from build123d import *

# Parameters (mm, degrees)
SZKIC1_W                     = 53
SZKIC1_H                     = 374
SZKIC1_W_2                   = 24
SZKIC1_H_2                   = 365
DODANIE_WYCI_GNI_CIE2_DEPTH  = 12
SZKIC2_W                     = 12
SZKIC2_H                     = 3.5
WYTNIJ_WYCI_GNI_CIE1_DEPTH   = 2
SZKIC3_W                     = 53
SZKIC3_H                     = 374
DODANIE_WYCI_GNI_CIE3_DEPTH  = 2
SZKIC4_W                     = 13.3
SZKIC4_H                     = 30.500081729
SZKIC4_W_2                   = 9.4
SZKIC4_H_2                   = 64.96
WYTNIJ_WYCI_GNI_CIE2_DEPTH   = 2
SZKIC5_W                     = 2
SZKIC5_H                     = 374
DODANIE_WYCI_GNI_CIE4_DEPTH  = 43
DODANIE_WYCI_GNI_CIE5_DEPTH  = 41.5
SZKIC7_W                     = 25.5
SZKIC7_H                     = 38.500081729
DODANIE_WYCI_GNI_CIE6_DEPTH  = 1.5
DODANIE_WYCI_GNI_CIE7_DEPTH  = 43
DODANIE_WYCI_GNI_CIE8_DEPTH  = 43
SZKIC15_W                    = 57
SZKIC15_H                    = 374
DODANIE_WYCI_GNI_CIE10_DEPTH = 1
SZKIC16_W                    = 57
SZKIC16_H                    = 374
DODANIE_WYCI_GNI_CIE11_DEPTH = 1
SZKIC17_W                    = 55
SZKIC17_H                    = 57
SZKIC17_W_2                  = 24
SZKIC17_H_2                  = 41.5
DODANIE_WYCI_GNI_CIE12_DEPTH = 1
SZKIC18_W                    = 55
SZKIC18_H                    = 57
DODANIE_WYCI_GNI_CIE13_DEPTH = 1
SZKIC19_W                    = 55
SZKIC19_H                    = 376
SZKIC19_W_2                  = 52
SZKIC19_H_2                  = 373
WYTNIJ_WYCI_GNI_CIE7_DEPTH   = 6
SZKIC23_W                    = 24
SZKIC23_H                    = 38.000081729
WYTNIJ_WYCI_GNI_CIE11_DEPTH  = 10
DODANIE_WYCI_GNI_CIE14_DEPTH = 32
SZKIC25_W                    = 24
SZKIC25_H                    = 2
DODANIE_WYCI_GNI_CIE15_DEPTH = 38
SZKIC27_R                    = 7
WYTNIJ_WYCI_GNI_CIE12_DEPTH  = 10
SZKIC29_W                    = 20
SZKIC29_H                    = 35.5
WYTNIJ_WYCI_GNI_CIE13_DEPTH  = 3
DODANIE_WYCI_GNI_CIE16_DEPTH = 6
SZKIC31_W                    = 24
SZKIC31_H                    = 2
DODANIE_WYCI_GNI_CIE17_DEPTH = 38
SZKIC32_R                    = 12.5
WYTNIJ_WYCI_GNI_CIE14_DEPTH  = 3
SZKIC33_W                    = 24
SZKIC33_H                    = 73
SZKIC33_H_2                  = 47
DODANIE_WYCI_GNI_CIE18_DEPTH = 5.5
SZKIC34_W                    = 55
SZKIC34_H                    = 51
DODANIE_WYCI_GNI_CIE19_DEPTH = 5.5
SZKIC35_W                    = 20
SZKIC35_H                    = 36
DODANIE_WYCI_GNI_CIE20_DEPTH = 1
SZKIC36_R                    = 12.5
DODANIE_WYCI_GNI_CIE21_DEPTH = 1
SZKIC37_W                    = 57
SZKIC37_H                    = 341.999918271
WYTNIJ_WYCI_GNI_CIE15_DEPTH  = 0.85


with BuildPart() as part:
    # Szkic1 → Dodanie-wyciągnięcie2 (new body)
    with BuildSketch(Plane.XY):
        with Locations((-65.426891924, -133.239080048)):
            Rectangle(SZKIC1_W, SZKIC1_H)
        with Locations((-78.426891924, -133.239080048)):
            Rectangle(SZKIC1_W_2, SZKIC1_H_2, mode=Mode.SUBTRACT)
        with Locations((-52.426891924, -133.239080048)):
            Rectangle(SZKIC1_W_2, SZKIC1_H_2, mode=Mode.SUBTRACT)
    extrude(amount=DODANIE_WYCI_GNI_CIE2_DEPTH)

    # Szkic2 → Wytnij-wyciągnięcie1 (cut)
    with BuildSketch(Plane.ZY.offset(66.426891924)):
        with Locations((6, 47.510919952)):
            Rectangle(SZKIC2_W, SZKIC2_H)
    extrude(amount=-WYTNIJ_WYCI_GNI_CIE1_DEPTH, mode=Mode.SUBTRACT)

    # Szkic3 → Dodanie-wyciągnięcie3 (add)
    with BuildSketch(Plane.XY.offset(12)):
        with Locations((-65.426891924, -133.239080048)):
            Rectangle(SZKIC3_W, SZKIC3_H)
    extrude(amount=DODANIE_WYCI_GNI_CIE3_DEPTH)

    # Szkic4 → Wytnij-wyciągnięcie2 (cut)
    with BuildSketch(Plane.XY.offset(14)):
        Polygon((-46.926891924, -11.039080048), (-56.326891924, -11.039080048), (-56.326891924, -35.399080048), (-56.326891924, -40.479080048), (-46.926891924, -40.479080048), (-46.926891924, -35.399080048), align=None)
        with Locations((-47.076891924, 34.010879088)):
            Rectangle(SZKIC4_W, SZKIC4_H)
        with Locations((-83.776891924, 34.010879088)):
            Rectangle(SZKIC4_W, SZKIC4_H)
        Polygon((-74.526891924, -35.399080048), (-74.526891924, -40.479080048), (-83.926891924, -40.479080048), (-83.926891924, -35.399080048), (-83.926891924, -11.039080048), (-74.526891924, -11.039080048), align=None)
        with Locations((-51.626891924, -133.719080048)):
            Rectangle(SZKIC4_W_2, SZKIC4_H_2)
        with Locations((-79.226891924, -133.719080048)):
            Rectangle(SZKIC4_W_2, SZKIC4_H_2)
    extrude(amount=-WYTNIJ_WYCI_GNI_CIE2_DEPTH, mode=Mode.SUBTRACT)

    # Szkic5 → Dodanie-wyciągnięcie4 (add)
    with BuildSketch(Plane.XY.offset(14)):
        with Locations((-65.426891924, -133.239080048)):
            Rectangle(SZKIC5_W, SZKIC5_H)
    extrude(amount=DODANIE_WYCI_GNI_CIE4_DEPTH)

    # Szkic6 → Dodanie-wyciągnięcie5 (add)
    with BuildSketch(Plane.XY.offset(14)):
        Polygon((-64.426891924, 16.760838223), (-40.426891924, 16.760838223), (-40.426891924, 53.760919952), (-38.926891924, 53.760919952), (-38.926891924, 15.260838223), (-64.426891924, 15.260838223), align=None)
        Polygon((-90.426891924, 53.760919952), (-91.926891924, 53.760919952), (-91.926891924, 15.260838223), (-66.426891924, 15.260838223), (-66.426891924, 16.760838223), (-90.426891924, 16.760838223), align=None)
    extrude(amount=DODANIE_WYCI_GNI_CIE5_DEPTH)

    # Szkic7 → Dodanie-wyciągnięcie6 (add)
    with BuildSketch(Plane.XY.offset(55.5)):
        with Locations((-51.676891924, 34.510879088)):
            Rectangle(SZKIC7_W, SZKIC7_H)
        with Locations((-79.176891924, 34.510879088)):
            Rectangle(SZKIC7_W, SZKIC7_H)
    extrude(amount=DODANIE_WYCI_GNI_CIE6_DEPTH)

    # Szkic10 → Dodanie-wyciągnięcie7 (add)
    with BuildSketch(Plane.XY.offset(14)):
        Polygon((-91.926891924, 15.260838223), (-91.926891924, -320.239080048), (-66.426891924, -320.239080048), (-66.426891924, -315.739080048), (-90.426891924, -315.739080048), (-90.426891924, 15.260838223), align=None)
    extrude(amount=DODANIE_WYCI_GNI_CIE7_DEPTH)

    # Szkic11 → Dodanie-wyciągnięcie8 (add)
    with BuildSketch(Plane.XY.offset(14)):
        Polygon((-38.926891924, 15.260838223), (-38.926891924, -320.239080048), (-64.426891924, -320.239080048), (-64.426891924, -315.739080048), (-40.426891924, -315.739080048), (-40.426891924, 15.260838223), align=None)
    extrude(amount=DODANIE_WYCI_GNI_CIE8_DEPTH)

    # Szkic15 → Dodanie-wyciągnięcie10 (add)
    with BuildSketch(Plane.ZY.offset(91.926891924)):
        with Locations((28.5, -133.239080048)):
            Rectangle(SZKIC15_W, SZKIC15_H)
    extrude(amount=DODANIE_WYCI_GNI_CIE10_DEPTH)

    # Szkic16 → Dodanie-wyciągnięcie11 (add)
    with BuildSketch(Plane(origin=(-38.926891924, 0, 0), x_dir=(0, 0, -1), z_dir=(1, 0, 0))):
        with Locations((-28.5, -133.239080048)):
            Rectangle(SZKIC16_W, SZKIC16_H)
    extrude(amount=DODANIE_WYCI_GNI_CIE11_DEPTH)

    # Szkic17 → Dodanie-wyciągnięcie12 (add)
    with BuildSketch(Plane(origin=(0, 53.760919952, 0), x_dir=(1, 0, 0), z_dir=(0, 1, 0))):
        with Locations((-65.426891924, -28.5)):
            Rectangle(SZKIC17_W, SZKIC17_H)
        with Locations((-52.426891924, -34.75)):
            Rectangle(SZKIC17_W_2, SZKIC17_H_2, mode=Mode.SUBTRACT)
        with Locations((-78.426891924, -34.75)):
            Rectangle(SZKIC17_W_2, SZKIC17_H_2, mode=Mode.SUBTRACT)
    extrude(amount=DODANIE_WYCI_GNI_CIE12_DEPTH)

    # Szkic18 → Dodanie-wyciągnięcie13 (add)
    with BuildSketch(Plane.XZ.offset(320.239080048)):
        with Locations((-65.426891924, 28.5)):
            Rectangle(SZKIC18_W, SZKIC18_H)
    extrude(amount=DODANIE_WYCI_GNI_CIE13_DEPTH)

    # Szkic19 → Wytnij-wyciągnięcie7 (cut)
    with BuildSketch(Plane(origin=(0, 0, 0), x_dir=(-1, 0, 0), z_dir=(0, 0, -1))):
        with Locations((65.426891924, -133.239080048)):
            Rectangle(SZKIC19_W, SZKIC19_H)
        with Locations((65.426891924, -133.239080048)):
            Rectangle(SZKIC19_W_2, SZKIC19_H_2, mode=Mode.SUBTRACT)
    extrude(amount=-WYTNIJ_WYCI_GNI_CIE7_DEPTH, mode=Mode.SUBTRACT)

    # Szkic23 → Wytnij-wyciągnięcie11 (cut)
    with BuildSketch(Plane.XY.offset(57)):
        with Locations((-52.426891924, 35.760879088)):
            Rectangle(SZKIC23_W, SZKIC23_H)
        with Locations((-78.426891924, 35.760879088)):
            Rectangle(SZKIC23_W, SZKIC23_H)
    extrude(amount=-WYTNIJ_WYCI_GNI_CIE11_DEPTH, mode=Mode.SUBTRACT)

    # Szkic24 → Dodanie-wyciągnięcie14 (add)
    with BuildSketch(Plane.XY.offset(57)):
        Polygon((-40.426891924, 54.760919952), (-37.926891924, 54.760919952), (-37.926891924, 15.260838223), (-66.426891924, 15.260838223), (-66.426891924, 16.760838223), (-66.426891924, 54.760919952), (-64.426891924, 54.760919952), (-64.426891924, 16.760838223), (-40.426891924, 16.760838223), align=None)
    extrude(amount=DODANIE_WYCI_GNI_CIE14_DEPTH)

    # Szkic25 → Dodanie-wyciągnięcie15 (add)
    with BuildSketch(Plane(origin=(0, 16.760838223, 0), x_dir=(1, 0, 0), z_dir=(0, 1, 0))):
        with Locations((-52.426891924, -88)):
            Rectangle(SZKIC25_W, SZKIC25_H)
    extrude(amount=DODANIE_WYCI_GNI_CIE15_DEPTH)

    # Szkic27 → Wytnij-wyciągnięcie12 (cut)
    with BuildSketch(Plane.XZ.offset(-15.260838223)):
        with Locations((-52.676891924, 78)):
            Circle(SZKIC27_R)
    extrude(amount=-WYTNIJ_WYCI_GNI_CIE12_DEPTH, mode=Mode.SUBTRACT)

    # Szkic29 → Wytnij-wyciągnięcie13 (cut)
    with BuildSketch(Plane(origin=(-37.926891924, 0, 0), x_dir=(0, 0, -1), z_dir=(1, 0, 0))):
        with Locations((-77, 35.010838223)):
            Rectangle(SZKIC29_W, SZKIC29_H)
    extrude(amount=-WYTNIJ_WYCI_GNI_CIE13_DEPTH, mode=Mode.SUBTRACT)

    # Szkic30 → Dodanie-wyciągnięcie16 (add)
    with BuildSketch(Plane.XY.offset(57)):
        Polygon((-66.426891924, 16.760838223), (-66.426891924, 15.260838223), (-92.926891924, 15.260838223), (-92.926891924, 54.760919952), (-90.426891924, 54.760919952), (-90.426891924, 16.760838223), align=None)
    extrude(amount=DODANIE_WYCI_GNI_CIE16_DEPTH)

    # Szkic31 → Dodanie-wyciągnięcie17 (add)
    with BuildSketch(Plane(origin=(0, 16.760838223, 0), x_dir=(1, 0, 0), z_dir=(0, 1, 0))):
        with Locations((-78.426891924, -62)):
            Rectangle(SZKIC31_W, SZKIC31_H)
    extrude(amount=DODANIE_WYCI_GNI_CIE17_DEPTH)

    # Szkic32 → Wytnij-wyciągnięcie14 (cut)
    with BuildSketch(Plane.ZY.offset(92.926891924)):
        with Locations((41, 33.010879088)):
            Circle(SZKIC32_R)
    extrude(amount=-WYTNIJ_WYCI_GNI_CIE14_DEPTH, mode=Mode.SUBTRACT)

    # Szkic33 → Dodanie-wyciągnięcie18 (add)
    with BuildSketch(Plane(origin=(0, 54.760919952, 0), x_dir=(1, 0, 0), z_dir=(0, 1, 0))):
        Polygon((-37.926891924, -89), (-66.426891924, -89), (-66.426891924, -63), (-92.926891924, -63), (-92.926891924, -6), (-37.926891924, -6), align=None)
        with Locations((-52.426891924, -50.5)):
            Rectangle(SZKIC33_W, SZKIC33_H, mode=Mode.SUBTRACT)
        with Locations((-78.426891924, -37.5)):
            Rectangle(SZKIC33_W, SZKIC33_H_2, mode=Mode.SUBTRACT)
    extrude(amount=DODANIE_WYCI_GNI_CIE18_DEPTH)

    # Szkic34 → Dodanie-wyciągnięcie19 (add)
    with BuildSketch(Plane.XZ.offset(321.239080048)):
        with Locations((-65.426891924, 31.5)):
            Rectangle(SZKIC34_W, SZKIC34_H)
    extrude(amount=DODANIE_WYCI_GNI_CIE19_DEPTH)

    # Szkic35 → Dodanie-wyciągnięcie20 (add)
    with BuildSketch(Plane(origin=(-37.926891924, 0, 0), x_dir=(0, 0, -1), z_dir=(1, 0, 0))):
        Polygon((-57, -326.739080048), (-57, 15.260838223), (-89, 15.260838223), (-89, 60.260919952), (-6, 60.260919952), (-6, -326.739080048), align=None)
        with Locations((-77, 34.760838223)):
            Rectangle(SZKIC35_W, SZKIC35_H, mode=Mode.SUBTRACT)
    extrude(amount=DODANIE_WYCI_GNI_CIE20_DEPTH)

    # Szkic36 → Dodanie-wyciągnięcie21 (add)
    with BuildSketch(Plane.ZY.offset(92.926891924)):
        Polygon((63, 60.260919952), (63, 15.260838223), (57, 15.260838223), (57, -326.739080048), (6, -326.739080048), (6, 60.260919952), align=None)
        with Locations((41, 33.010879088)):
            Circle(SZKIC36_R, mode=Mode.SUBTRACT)
    extrude(amount=DODANIE_WYCI_GNI_CIE21_DEPTH)

    # Szkic37 → Wytnij-wyciągnięcie15 (cut)
    with BuildSketch(Plane.XY.offset(57)):
        with Locations((-65.426891924, -155.739120912)):
            Rectangle(SZKIC37_W, SZKIC37_H)
    extrude(amount=-WYTNIJ_WYCI_GNI_CIE15_DEPTH, mode=Mode.SUBTRACT)


solid = part.part
Work out the finished part from the listing and answer in its coordinate system (mm). A direction names the side the tool comes from. Round coordinates to 2 decimals unless told otherwise and drop trailing zeros. Write each loop counter-clockwise with the first axis right and the second up, starting at its lowest first coordinate (ties: lowest second). Pieces come first, ordered by that corner, then holes.
1) A cutting plane is placed at A-A (z = 78). Give the vertices of the cut face in (x, y), plus the area to 3 significant figures.
2) The mould has two halves that part along Y. Classify faces 1 (the flat face through (-64.427, -138, 6)), 2 (the flat face through (-65, 60.261, 35)), 3 (the flat face through (-52, 37, 89)): pulls with the +Y half, pulls with the -Y half, needs draft (parallel to the pull), parting line crosses it, or undercut.
3) A cutting plane is placed at D-D (y = -175.5). Give the vertices of the cut face in (x, z).
4) Given pin 1 Ø4 at (x, y) = (-86, -264.5) entering from +Z; pin 2 Ø1 at (x, z) = (-38.5, 78.5) entering from -Y; pin 3 Ø14 at (x, y) = (-75, 44) entering from +Z, each flat-ended and moving along its own axis, determine where each tip first touches the part or whether it passes through.
5) A cutting plane is placed at B-B (y = -19). Give the number of separate pieces and of enclosed holes in the cut face, plus the area to 3 significant figures.
6) A cutting plane is placed at C-C (z = 41). Give the vertices of the cut face in (x, y).
7) Straight lines are drawn through the part: line 1 (X direction, y = -116.5, z = 34); line 2 (Y direction, x = -93, z = 41); line 3 (Y direction, x = -46, z = 4.5). For each, find the intervals that lie inside material, in ascending order.
8) A tool of negligible diameter and unlimited length cuts with its end or side. For faces 4 (the flat face through (-66.427, 37, 52)), 5 (the flat face through (-93.927, -131, 35)), 6 (the flat face through (-53, -315.739, 35)), 7 (the flat face through (-66.427, -138, 6)), from which of +Z, -Z, +X, -X, +Y, -Y can it reach the whole face along a straight path? Write none if from no direction.
Completed:
1. outline: (-66.43, 15.26) - (-59.68, 15.26) - (-59.68, 16.76) - (-64.43, 16.76) - (-64.43, 60.26) - (-66.43, 60.26) - close; (-45.68, 15.26) - (-36.93, 15.26) - (-36.93, 16.76) - (-37.93, 16.76) - (-37.93, 17.26) - (-40.43, 17.26) - (-40.43, 16.76) - (-45.68, 16.76) - close; (-40.43, 52.76) - (-36.93, 52.76) - (-36.93, 60.26) - (-40.43, 60.26) - close
1. area: 138 mm2
2. face 1: undercut
2. face 2: pulls with the +Y half
2. face 3: needs draft
3. outline: (-93.93, 6) - (-91.43, 6) - (-91.43, 0) - (-90.43, 0) - (-90.43, 12) - (-66.43, 12) - (-66.43, 0) - (-64.43, 0) - (-64.43, 12) - (-40.43, 12) - (-40.43, 0) - (-39.43, 0) - (-39.43, 6) - (-36.93, 6) - (-36.93, 56.15) - (-40.43, 56.15) - (-40.43, 14) - (-64.43, 14) - (-64.43, 56.15) - (-66.43, 56.15) - (-66.43, 14) - (-90.43, 14) - (-90.43, 56.15) - (-93.93, 56.15) - close
4. pin 1: stops at z = 14
4. pin 2: stops at y = 15.26
4. pin 3: stops at z = 63
5. separate pieces: 3
5. enclosed holes: 0
5. area: 534 mm2
6. outline: (-93.93, -326.74) - (-36.93, -326.74) - (-36.93, 60.26) - (-40.43, 60.26) - (-40.43, 16.76) - (-64.43, 16.76) - (-64.43, 60.26) - (-66.43, 60.26) - (-66.43, 16.76) - (-90.43, 16.76) - (-90.43, 20.51) - (-93.93, 20.51) - close; (-93.93, 45.51) - (-90.43, 45.51) - (-90.43, 60.26) - (-93.93, 60.26) - close; hole (-90.43, -315.74) - (-66.43, -315.74) - (-66.43, 15.26) - (-90.43, 15.26) - close; hole (-64.43, -315.74) - (-40.43, -315.74) - (-40.43, 15.26) - (-64.43, 15.26) - close
7. line 1: x = -93.93 to -90.43, -66.43 to -64.43, -40.43 to -36.93
7. line 2: y = -326.74 to 20.51, 45.51 to 60.26
7. line 3: y = -319.74 to -315.74, 49.26 to 53.26
8. face 4: +Y
8. face 5: +Z, -Z, -X, +Y, -Y
8. face 6: +Z
8. face 7: -Z
